Input: part model. Units: mm. Frame: model coordinates. A direction names the side the tool comes from. Round coordinates to 2 decimals unless told otherwise and drop trailing zeros. Loops run counter-clockwise (first coordinate to the right, second up) from the corner with the lowest first, then second, coordinate; pieces in that order, holes last.
1) Access query for faces 1 (the face through (10.631, -12.173, 2.465)), 2 (the face through (-14, -17, 1.6)). Directions: +Z, -Z, +X, -X, +Y, -Y. A direction counts if a zero-diameter tool reaches every point of the face in a straight line with its end or side. Return the directions, or none.
2) Draft query along X for faces 3 (the face through (0, -22.5, 2)), 4 (the face through (-22.5, 0, 2)), 5 (the face through (-18.722, 15.923, 3.276)). Return one class per face: pulls with the +X half, pulls with the -X half, needs draft (parallel to the pull), parting line crosses it, or undercut.
3) Section A-A, the plane y = 0. Return loops of the section in (x, z), and give its area (3 significant figures).
4) Section D-D, the plane y = 15.5. Return loops of the section in (x, z).
5) First-contact query: pin 1 (3 mm diameter, centred on x = 16.5, y = 15, fed in from +Z). Flat tip, straight axial feed; report the tip coordinate or a pass-through.
6) Section C-C, the plane z = 4.3. State how many separate pieces and enclosed holes the cut face has, and give its area (3 significant figures).
7) Ray query, line 1 along X through (y, z) = (15.5, 0.4); line 2 along Y through (x, z) = (-15.5, 4.1). Return the intervals inside material, ascending.
Autodesk Inventor part; units mm, degrees
ref_plane "YZ Plane" through (0, 0, 0) normal (1, 0, 0) x (0, 1, 0)
ref_plane "XZ Plane" through (0, 0, 0) normal (0, 1, 0) x (-1, 0, 0)
ref_plane "XY Plane" through (0, 0, 0) normal (0, 0, 1) x (1, 0, 0)
sketch "Skizze1" plane through (0, 0, 0) normal (0, 0, 1) x (1, 0, 0)
  line L0 (-22.5, 22.5) -> (22.5, 22.5)
  line L1 (22.5, 22.5) -> (22.5, -22.5)
  line L2 (22.5, -22.5) -> (-22.5, -22.5)
  line L3 (-22.5, -22.5) -> (-22.5, 22.5)
  circle A0 centre (0, 0) radius 11
  line L4 (-31.5, 0) -> (31.5, 0)
  line L5 (0, -31.5) -> (0, 31.5)
  dimension "d0" = 22
  dimension "d1" = 45
extrude "Extrusion1" add sketch "Skizze1" along normal blind 5 contours L0 L5 A0 L4 L3 | L0 L1 L4 A0 L5 | L4 A0 L5 L2 L3 | L1 L2 L5 A0 L4
sketch "Skizze2" plane through (0, 0, 5) normal (0, 0, 1) x (1, 0, 0)
  line L0 (-11, 11) -> (11, 11)
  line L1 (11, 11) -> (11, -11)
  line L2 (11, -11) -> (-11, -11)
  line L3 (-11, -11) -> (-11, 11)
  line L4 (-31.5, 0) -> (31.5, 0)
  line L5 (0, -31.5) -> (0, 31.5)
  dimension "d4" = 22
hole "Bohrung1" at (-11, 11, 5) at (11, 11, 5) at (11, -11, 5) at (-11, -11, 5) direction (0, 0, -1) diameter 2.459 end through all
sketch "Skizze3" plane through (0, 0, 5) normal (0, 0, 1) x (1, 0, 0)
  line L0 (-31.5, 0) -> (31.5, 0)
  line L1 (0, -31.5) -> (0, 31.5)
  line L2 (-15.5, 15.5) -> (15.5, 15.5)
  line L3 (15.5, 15.5) -> (15.5, -15.5)
  line L4 (15.5, -15.5) -> (-15.5, -15.5)
  line L5 (-15.5, -15.5) -> (-15.5, 15.5)
  dimension "d12" = 31
hole "Bohrung2" at (15.5, -15.5, 5) at (-15.5, 15.5, 5) at (15.5, 15.5, 5) at (-15.5, -15.5, 5) direction (0, 0, -1) diameter 3.4 end through all counterbore diameter 6.5 counterbore depth 3.4
properties part number "13_0204_060"
Final values:
1. face 1: +Z, -Z
1. face 2: +Z
2. face 3: needs draft
2. face 4: pulls with the -X half
2. face 5: undercut
3. outline: (-22.5, 0) - (-11, 0) - (-11, 5) - (-22.5, 5) - close; (11, 0) - (22.5, 0) - (22.5, 5) - (11, 5) - close
3. area: 115 mm2
4. outline: (-22.5, 0) - (-17.2, 0) - (-17.2, 1.6) - (-18.75, 1.6) - (-18.75, 5) - (-22.5, 5) - close; (-13.8, 0) - (13.8, 0) - (13.8, 1.6) - (12.25, 1.6) - (12.25, 5) - (-12.25, 5) - (-12.25, 1.6) - (-13.8, 1.6) - close; (17.2, 0) - (22.5, 0) - (22.5, 5) - (18.75, 5) - (18.75, 1.6) - (17.2, 1.6) - close
5. pin 1: stops at z = 1.6
6. separate pieces: 1
6. enclosed holes: 9
6. area: 1,490 mm2
7. line 1: x = -22.5 to -17.2, -13.8 to 13.8, 17.2 to 22.5
7. line 2: y = -22.5 to -18.75, -12.25 to 12.25, 18.75 to 22.5
